from build123d import *

# Parameters (mm, degrees)
BRIDA_BASE1_DEPTH       = 80
CROQUIS13_W             = 3
CROQUIS13_H             = 10
CROQUIS13_H_2           = 15
SALIENTE_EXTRUIR2_DEPTH = 3
CROQUIS14_W             = 3
CROQUIS14_H             = 10
CROQUIS14_H_2           = 15
SALIENTE_EXTRUIR3_DEPTH = 3
CORTAR_EXTRUIR1_DEPTH   = 10


# Sheet-metal steps are written as plain solids
with BuildPart() as part:
    # Croquis7 → Brida base1 (new body)
    with BuildSketch(Plane.XY):
        with BuildLine():
            Line((3, 29.270313854), (3, 0))
            Line((3, 0), (3, -89.088238126))
            ThreePointArc((3, -89.088238126), (3.301536896, -90.798338842), (4.169777784, -92.302176174))
            Line((4.169777784, -92.302176174), (21.58176162, -113.052970465))
            Line((21.58176162, -113.052970465), (19.283628291, -114.981333294))
            Line((19.283628291, -114.981333294), (1.871644455, -94.230539003))
            ThreePointArc((1.871644455, -94.230539003), (0.482459034, -91.824399272), (0, -89.088238126))
            Line((0, -89.088238126), (0, 0))
            Line((0, 0), (0, 29.270313854))
            Line((0, 29.270313854), (3, 29.270313854))
        make_face()
    extrude(amount=BRIDA_BASE1_DEPTH)

    # Croquis13 → Saliente-Extruir2 (add)
    with BuildSketch(Plane.XY.offset(80)):
        with Locations((1.5, -15.729686146)):
            Rectangle(CROQUIS13_W, CROQUIS13_H)
        Polygon((12.855752194, -107.320888862), (15.153885523, -105.392526033), (8.726009426, -97.732081602), (6.427876097, -99.660444431), align=None)
        with Locations((1.5, -43.229686146)):
            Rectangle(CROQUIS13_W, CROQUIS13_H_2)
        with Locations((1.5, -73.229686146)):
            Rectangle(CROQUIS13_W, CROQUIS13_H_2)
    extrude(amount=SALIENTE_EXTRUIR2_DEPTH)

    # Croquis14 → Saliente-Extruir3 (add)
    with BuildSketch(Plane(origin=(0, 0, 0), x_dir=(-1, 0, 0), z_dir=(0, 0, -1))):
        with Locations((-1.5, -15.729686146)):
            Rectangle(CROQUIS14_W, CROQUIS14_H)
        Polygon((-15.153885523, -105.392526033), (-12.855752194, -107.320888862), (-6.427876097, -99.660444431), (-8.726009426, -97.732081602), align=None)
        with Locations((-1.5, -43.229686146)):
            Rectangle(CROQUIS14_W, CROQUIS14_H_2)
        with Locations((-1.5, -73.229686146)):
            Rectangle(CROQUIS14_W, CROQUIS14_H_2)
    extrude(amount=SALIENTE_EXTRUIR3_DEPTH)

    # Croquis15 → Cortar-Extruir1 (cut)
    with BuildSketch(Plane.ZY):
        Polygon((8, 20.520313854), (0, 20.520313854), (0, 18.020313854), (8, 18.020313854), (8, 15.770313854), (11, 15.770313854), (11, 18.020313854), (15, 18.020313854), (15, 20.520313854), (11, 20.520313854), (11, 22.770313854), (8, 22.770313854), align=None)
        Polygon((80, 18.020313854), (80, 20.520313854), (72, 20.520313854), (72, 22.770313854), (69, 22.770313854), (69, 20.520313854), (65, 20.520313854), (65, 18.020313854), (69, 18.020313854), (69, 15.770313854), (72, 15.770313854), (72, 18.020313854), align=None)
        Polygon((54.5, 29.270313854), (51.5, 29.270313854), (51.5, 21.270313854), (49.5, 21.270313854), (49.5, 18.270313854), (51.5, 18.270313854), (51.5, 14.270313854), (54.5, 14.270313854), (54.5, 18.270313854), (56.5, 18.270313854), (56.5, 21.270313854), (54.5, 21.270313854), align=None)
        Polygon((28.5, 29.270313854), (25.5, 29.270313854), (25.5, 21.270313854), (23.5, 21.270313854), (23.5, 18.270313854), (25.5, 18.270313854), (25.5, 14.270313854), (28.5, 14.270313854), (28.5, 18.270313854), (30.5, 18.270313854), (30.5, 21.270313854), (28.5, 21.270313854), align=None)
    extrude(amount=-CORTAR_EXTRUIR1_DEPTH, mode=Mode.SUBTRACT)


solid = part.part
Part model, mm, in its own coordinate system. A direction names the side the tool comes from. Round coordinates to 2 decimals unless told otherwise and drop trailing zeros. Loops run counter-clockwise (first coordinate to the right, second up) from the corner with the lowest first, then second, coordinate; pieces in that order, holes last. Notation, with made-up numbers: (1.5, 58.25) - (9.5, 58.25) arc R10 ccw to (9.5, 64.25) - close; hole circle Ø5 at (83, 67.5). An arc over 180 degrees is marked (long way). Answer as a JSON object with one key per item and string values.
Item 1: Tool access for faces 5 (the face through (1, 20.52, 4)), 6 (the face through (1, 20.52, 76)), 7 (the face through (1, -80.73, 81)), 8 (the face through (1, 20, 49.5)), 9 (the face through (1, 25, 28.5)): list every direction of +Z, -Z, +X, -X, +Y, -Y with a clear straight run to the whole face (end or side of a thin tool).
Output:
{"face 5": "-Z, +X, -X", "face 6": "+Z, +X, -X", "face 7": "+Z, +X, -X, -Y", "face 8": "+X, -X", "face 9": "+X, -X, +Y"}
Item 2: Wall check: L1, parallel to X at y = -51.5, z = 39; L2, parallel to Y at x = 1, z = 58; L3, parallel to Y at x = 13.5, z = 72. Give the ranges that are in metal, low to high.
Output:
{"L1": "0 to 3", "L2": "-92.96 to 29.27", "L3": "-108.09 to -103.42"}
Item 3: Pin check, flat tips, straight feed: pin 1 (1.6 mm diameter, centred on x = 1, z = 25, fed in from -Y); pin 2 (1.5 mm diameter, centred on x = 2, y = -26.5, fed in from -Z); pin 3 (12 mm diameter, centred on x = 7, y = 8, fed in from +Z). Stop position of each tip, or through.
Output:
{"pin 1": "y = -94.14", "pin 2": "z = 0", "pin 3": "z = 80"}
Item 4: Band-saw the part on A-A on z = 77. List the corners of the cut face in (x, y).
Output:
{"outline": "(0, -89.09) arc R8 ccw to (1.87, -94.23) - (19.28, -114.98) - (21.58, -113.05) - (4.17, -92.3) arc R5 cw to (3, -89.09) - (3, 18.02) - (0, 18.02) - close; (0, 20.52) - (3, 20.52) - (3, 29.27) - (0, 29.27) - close"}
Item 5: Pull direction Y, two halves, no side cores. Call faces 1 (the face through (2.8, -89.4, 80)), 2 (the face through (3.293, -90.775, 39.44)), 3 (the face through (1, -20.73, 81)), 4 (the face through (2, -50.73, -1)): pulls with the +Y half, pulls with the -Y half, needs draft (parallel to the pull), parting line crosses it, or undercut.
Output:
{"face 1": "needs draft", "face 2": "pulls with the +Y half", "face 3": "undercut", "face 4": "undercut"}
Item 6: Band-saw the part on C-C on y = -40. List the corners of the cut face in (x, z).
Output:
{"outline": "(0, -3) - (3, -3) - (3, 83) - (0, 83) - close"}
Item 7: Band-saw the part on D-D on x = 17.75. List the corners of the cut face in (y, z).
Output:
{"outline": "(-113.15, 0) - (-108.49, 0) - (-108.49, 80) - (-113.15, 80) - close"}
Item 8: Band-saw the part on B-B on z = 21. List the corners of the cut face in (x, y), plus the area to 3 significant figures.
Output:
{"outline": "(0, -89.09) arc R8 ccw to (1.87, -94.23) - (19.28, -114.98) - (21.58, -113.05) - (4.17, -92.3) arc R5 cw to (3, -89.09) - (3, 29.27) - (0, 29.27) - close", "area": "450 mm2"}
